from build123d import *

# Parameters (mm, degrees)
F0_W     = 40.5
F0_H     = 19
F0_R     = 2.6
F1_DEPTH = 1.6
F0_W_2   = 19
F0_H_2   = 40.5
F0_R_2   = 1.5
F2_DEPTH = 3.2
F3_DEPTH = 1.6


with BuildPart() as f1:
    # F0 (on Top) → F1 (new body)
    with BuildSketch(Plane.XY):
        with Locations((-29.75, 0)):
            Rectangle(F0_W, F0_H)
        with Locations((-45, 0)):
            Circle(F0_R, mode=Mode.SUBTRACT)
    extrude(amount=F1_DEPTH)



with BuildPart() as f1b:
    # F0 (on Top) → F1, piece 2 (new body)
    with BuildSketch(Plane.XY):
        with Locations((0, 29.75)):
            Rectangle(F0_W_2, F0_H_2)
        with Locations((0, 45)):
            Circle(F0_R, mode=Mode.SUBTRACT)
    extrude(amount=F1_DEPTH)


with BuildPart() as f1c:
    # F0 (on Top) → F1, piece 3 (new body)
    with BuildSketch(Plane.XY):
        with Locations((29.75, 0)):
            Rectangle(F0_W, F0_H)
        with Locations((45, 0)):
            Circle(F0_R, mode=Mode.SUBTRACT)
    extrude(amount=F1_DEPTH)


with BuildPart() as f1d:
    # F0 (on Top) → F1, piece 4 (new body)
    with BuildSketch(Plane.XY):
        with Locations((0, -29.75)):
            Rectangle(F0_W_2, F0_H_2)
        with Locations((0, -45)):
            Circle(F0_R, mode=Mode.SUBTRACT)
    extrude(amount=F1_DEPTH)


with BuildPart() as f1_1:
    add(f1.part)

    add(f1b.part)  # F2 merges F1b

    add(f1c.part)  # F2 merges F1c

    add(f1d.part)  # F2 merges F1d
    # F0 (on Top) → F2 (join)
    with BuildSketch(Plane.XY):
        Rectangle(F0_W_2, F0_H)
        with Locations((-6, -6)):
            Circle(F0_R_2, mode=Mode.SUBTRACT)
        with Locations((6, -6)):
            Circle(F0_R_2, mode=Mode.SUBTRACT)
        with Locations((-6, 6)):
            Circle(F0_R_2, mode=Mode.SUBTRACT)
        with Locations((6, 6)):
            Circle(F0_R_2, mode=Mode.SUBTRACT)
    extrude(amount=F2_DEPTH)

    # F0 (on Top) → F3 (join)
    with BuildSketch(Plane.XY):
        with Locations((6, -6)):
            Circle(F0_R_2)
        with Locations((6, 6)):
            Circle(F0_R_2)
        with Locations((-6, 6)):
            Circle(F0_R_2)
        with Locations((-6, -6)):
            Circle(F0_R_2)
    extrude(amount=F3_DEPTH)


solid = f1_1.part
Geometry: final body of the model. Coordinates: model frame, mm. A direction names the side the tool comes from. Give positions to 0.01 mm unless a question says otherwise; leave off trailing zeros. Write each loop counter-clockwise with the first axis right and the second up, starting at its lowest first coordinate (ties: lowest second). Pieces come first, ordered by that corner, then holes. Notation, with made-up numbers: (54, 7.25) -> (83, 7.25) arc R30 cw to (83, 38.25) -> close; hole circle Ø5 at (15, 24.25). An arc over 180 degrees is marked (long way). Answer as a JSON object with one key per item and string values.
1. Ray query, probe 1 along Y at (x, z) = (-6, 2.2); probe 2 along Y at (x, z) = (0, 0.65); probe 3 along Y at (x, z) = (40, 0.75). Return the intervals inside material, ascending. Write a range as from..to.
Ans:
{"probe 1": "y = -9.5..-7.5, -4.5..4.5, 7.5..9.5", "probe 2": "y = -50..-47.6, -42.4..42.4, 47.6..50", "probe 3": "y = -9.5..9.5"}
2. Access query for faces 3 (the flat face through (0, 30, 1.6)), 4 (the flat face through (29, 0, 1.6)), 5 (the flat face through (-30, 0, 1.6)), 6 (the cylindrical face through (4.8, 5.1, 2.4)), 7 (the flat face through (0, -29, 1.6)). Directions: +Z, -Z, +X, -X, +Y, -Y. A direction counts if a zero-diameter tool reaches every point of the face in a straight line with its end or side. Return the directions, or none.
Ans:
{"face 3": "+Z, +X, -X, +Y", "face 4": "+Z, +X, +Y, -Y", "face 5": "+Z, -X, +Y, -Y", "face 6": "+Z", "face 7": "+Z, +X, -X, -Y"}
3. Cut plane B-B on y = -45. Output: boundary loops of the cut face in (x, z).
Ans:
{"outline": "(-9.5, 0) -> (-2.6, 0) -> (-2.6, 1.6) -> (-9.5, 1.6) -> close; (2.6, 0) -> (9.5, 0) -> (9.5, 1.6) -> (2.6, 1.6) -> close"}
4. Mould query, pull axis Y, two halves, no side actions, for faces 1 (the flat face through (0, 0, 3.2)), 2 (the cylindrical face through (-7.2, 5.1, 2.4)). Classes: pulls with the +Y half, pulls with the -Y half, needs draft (parallel to the pull), parting line crosses it, or undercut.
Ans:
{"face 1": "needs draft", "face 2": "undercut"}
5. Cut plane A-A on x = 0. Output: boundary loops of the cut face in (y, z), and give its area (3 significant figures).
Ans:
{"outline": "(-50, 0) -> (-47.6, 0) -> (-47.6, 1.6) -> (-50, 1.6) -> close; (-42.4, 0) -> (42.4, 0) -> (42.4, 1.6) -> (9.5, 1.6) -> (9.5, 3.2) -> (-9.5, 3.2) -> (-9.5, 1.6) -> (-42.4, 1.6) -> close; (47.6, 0) -> (50, 0) -> (50, 1.6) -> (47.6, 1.6) -> close", "area": "174 mm^2"}
6. Cut plane D-D on y = 6. Output: boundary loops of the cut face in (x, z).
Ans:
{"outline": "(-50, 0) -> (50, 0) -> (50, 1.6) -> (9.5, 1.6) -> (9.5, 3.2) -> (7.5, 3.2) -> (7.5, 1.6) -> (4.5, 1.6) -> (4.5, 3.2) -> (-4.5, 3.2) -> (-4.5, 1.6) -> (-7.5, 1.6) -> (-7.5, 3.2) -> (-9.5, 3.2) -> (-9.5, 1.6) -> (-50, 1.6) -> close"}
7. Contact query for flat-ended pins moving along their axis: pin 1 (2.5 mm diameter, centred on x = -6, y = -6, fed in from +Z); pin 2 (4 mm diameter, centred on x = 45, y = 0, fed in from -Z); pin 3 (1.3 mm diameter, centred on y = -20.5, z = 0.5, fed in from -X); pin 4 (1 mm diameter, centred on x = -31, z = 0.5, fed in from -Y). Output: stop coordinate, or through.
Ans:
{"pin 1": "stops at z = 1.6", "pin 2": "passes through", "pin 3": "stops at x = -9.5", "pin 4": "stops at y = -9.5"}
8. Cut plane C-C on z = 0.5. Output: boundary loops of the cut face in (x, y).
Ans:
{"outline": "(-50, -9.5) -> (-9.5, -9.5) -> (-9.5, -50) -> (9.5, -50) -> (9.5, -9.5) -> (50, -9.5) -> (50, 9.5) -> (9.5, 9.5) -> (9.5, 50) -> (-9.5, 50) -> (-9.5, 9.5) -> (-50, 9.5) -> close; hole circle Ø5.2 at (-45, 0); hole circle Ø5.2 at (0, -45); hole circle Ø5.2 at (0, 45); hole circle Ø5.2 at (45, 0)"}
